from build123d import *

# Parameters (mm, degrees)
F2_R      = 5
F0_R      = 3.5
F4_R      = 2
F3_FACE_R = 5
F6_R      = 5
F7_FACE_R = 5
F9_R      = 2.5
F11_R     = 2


with BuildPart() as f3:
    # F2 (on offset) → F3 section 0
    with BuildSketch(Plane.XY.offset(45)):
        Circle(F2_R)
    # F0 (on Top) → F3 section 1
    with BuildSketch(Plane.XY):
        Circle(F0_R)
    loft()

    # F4
    f4_edges = [f3.edges().sort_by_distance(p)[0] for p in [
        (-3.5, 0, 0),
    ]]
    fillet(f4_edges, radius=F4_R)

    # F3_face (on face) → F7 section 0
    with BuildSketch(Plane.XY.offset(45)):
        Circle(F3_FACE_R)
    # F6 (on offset) → F7 section 1
    with BuildSketch(Plane.XY.offset(65)):
        Circle(F6_R)
    loft()

    # F7_face (on face) → F10 section 0
    with BuildSketch(Plane.XY.offset(65)):
        Circle(F7_FACE_R)
    # F9 (on offset) → F10 section 1
    with BuildSketch(Plane.XY.offset(140)):
        Circle(F9_R)
    loft()

    # F11
    f11_edges = [f3.edges().sort_by_distance(p)[0] for p in [
        (-2.5, 0, 140),
    ]]
    fillet(f11_edges, radius=F11_R)


solid = f3.part
Can you work these out from the model? Positions are in its coordinate system, mm. A direction names the side the tool comes from. Round coordinates to 2 decimals unless told otherwise and drop trailing zeros. Write each loop counter-clockwise with the first axis right and the second up, starting at its lowest first coordinate (ties: lowest second). Pieces come first, ordered by that corner, then holes. Notation, with made-up numbers: M -28.75,84 L 20.25,84 A14 ccw 20.25,92 Z; hole C 40,23 d4. An arc over 180 degrees is marked long. Use CSV: the item, a comma, the result in double quotes.
(1) Imagine slicing it at B-B (z = 93). Write out the boundary of the cut face in (x, y).
Check values:
outline,"C 0,0 d8.13"
(2) I'm going to push flat-ended pins straight in: pin 1 (2 mm diameter, centred on x = -2.5, z = 70, fed in from -Y); pin 2 (4 mm diameter, centred on x = 3.5, y = -2.5, fed in from +Z); pin 3 (6 mm diameter, centred on x = -3, z = 89.5, fed in from -Y). Where does each tip first touch, or does it pass through?
Check values:
pin 1,"y = -4.6"
pin 2,"z = 138.99"
pin 3,"y = -4.22"
(3) Imagine slicing it at A-A (z = 108.5). Write out the boundary of the cut face in (x, y), plus the area to 3 significant figures.
Check values:
outline,"C 0,0 d7.1"
area,"39.6 mm^2"
(4) I need wall thicknesses on line 1 along Y through (x, z) = (-1, 133); line 2 along X through (y, z) = (1.75, 14); line 3 along Y through (x, z) = (0.5, 53.5). Which ranges of each line are inside material? Lowest first, please.
Check values:
line 1,"-2.54 to 2.54"
line 2,"-3.56 to 3.56"
line 3,"-4.97 to 4.97"
(5) On a 3-axis mill with a long thin cutter (end or side, diameter ignored), from which of +Z, -Z, +X, -X, +Y, -Y can I reach the whole of each face in a straight line? I mean faces 1 (the conical face through (-2.99, -2.29, 102.04)), 2 (the flat face through (0, 0, 0)), 3 (the conical face through (4.075, 1.283, 23.165)). Say none if no direction works.
Check values:
face 1,"+Z"
face 2,"-Z, +X, -X, +Y, -Y"
face 3,"-Z"
